from build123d import *

# Parameters (mm, degrees)
F0_W     = 165.1
F0_H     = 38.1
F1_DEPTH = 12.7
F2_R     = 25.4
F3_DEPTH = 101.6
F4_R     = 19.05
F5_DEPTH = 76.2


with BuildPart() as f1:
    # F0 (on Front) → F1 (new body)
    with BuildSketch(Plane.XZ):
        Rectangle(F0_W, F0_H)
    extrude(amount=F1_DEPTH)

    # F2 (on Front) → F3 (join)
    with BuildSketch(Plane.XZ):
        Circle(F2_R)
    extrude(amount=F3_DEPTH)

    # F4 (on Front) → F5 (join)
    with BuildSketch(Plane.XZ):
        with Locations((56.968745, 0)):
            Circle(F4_R)
        with Locations((-56.4654, 0)):
            Circle(F4_R)
        Circle(F4_R)
    extrude(amount=-F5_DEPTH)


solid = f1.part
The listing builds one solid part. Answer for the finished solid, in the listing's coordinates (mm). A direction names the side the tool comes from. Coordinates: 2 decimals unless noted, no trailing zeros. Write each loop counter-clockwise with the first axis right and the second up, starting at its lowest first coordinate (ties: lowest second). Pieces come first, ordered by that corner, then holes. Notation, with made-up numbers: M 47.5,-17.75 L 95.5,-17.75 A17 ccw 95.5,-2.75 Z; hole C -35,86 d1. An arc over 180 degrees is marked long. Use one line per item in the form item = value.
Item 1: The mould has two halves that part along X. Classify faces 1 (the face through (-50, -6, -19.05)), 2 (the face through (82.55, -6, 0)), 3 (the face through (74.566, 37.567, -7.296)): released by +X, released by -X, zero draft, split by the parting line, or undercut.
Model answer:
face_1 = zero draft
face_2 = released by +X
face_3 = undercut
Item 2: Find section A-A, the plane z = 0. Give the vertices of the cut face in (x, y), plus the area to 3 significant figures.
Model answer:
outline = M -82.55,-12.7 L -25.4,-12.7 L -25.4,-101.6 L 25.4,-101.6 L 25.4,-12.7 L 82.55,-12.7 L 82.55,0 L 76.02,0 L 76.02,76.2 L 37.92,76.2 L 37.92,0 L 19.05,0 L 19.05,76.2 L -19.05,76.2 L -19.05,0 L -37.42,0 L -37.42,76.2 L -75.52,76.2 L -75.52,0 L -82.55,0 Z
area = 15,300 mm2
Item 3: For faces 4 (the face through (49, -6, -19.05)), 5 (the face through (78, 0, 0)), 6 (the face through (-78, 0, 0)), 7 (the face through (24.227, -50.089, 7.629)), 8 (the face through (-50, -6, 19.05)), determine the directions among +Z, -Z, +X, -X, +Y, -Y from which every point of the face is accessible in a straight line to the end or side of a thin tool.
Model answer:
face_4 = -Z, +X, +Y, -Y
face_5 = +X, +Y
face_6 = -X, +Y
face_7 = -Y
face_8 = +Z, -X, +Y, -Y
Item 4: Find section B-B, the plane y = 62. Give the vertices of the cut face in (x, z), plus the area to 3 significant figures.
Model answer:
outline = C -56.47,0 d38.1; C 0,0 d38.1; C 56.97,0 d38.1
area = 3,420 mm2
Item 5: Find the intervals of material crossed by probe 1 along X at (y, z) = (43, -13); probe 2 along X at (y, z) = (23.5, 17.5); probe 3 along Y at (x, z) = (-45, 3.5), in increasing order.
Model answer:
probe_1 = -70.39 to -42.54, -13.92 to 13.92, 43.04 to 70.89
probe_2 = -63.99 to -48.94, -7.53 to 7.53, 49.44 to 64.5
probe_3 = -12.7 to 76.2
Item 6: Find section D-D, the plane x = -40. Give the vertices of the cut face in (y, z), plus the area to 3 significant figures.
Model answer:
outline = M -12.7,-19.05 L 0,-19.05 L 0,-9.58 L 76.2,-9.58 L 76.2,9.58 L 0,9.58 L 0,19.05 L -12.7,19.05 Z
area = 1,940 mm2
Item 7: Find section C-C, the plane x = 0. Give the vertices of the cut face in (y, z).
Model answer:
outline = M -101.6,-25.4 L 0,-25.4 L 0,-19.05 L 76.2,-19.05 L 76.2,19.05 L 0,19.05 L 0,25.4 L -101.6,25.4 Z
Item 8: Given P1, Ø8, axis at y = 6.5, z = 18, coming from the +X side; P2, Ø3, axis at x = -40.5, z = -10, coming from the -Y side; P3, Ø6, axis at x = -5.5, y = 43, coming from the +Z side, each flat-ended and moving along its own axis, determine where each tip first touches the part or whether it passes through.
Model answer:
P1 = 69.89
P2 = -12.7
P3 = 18.89
